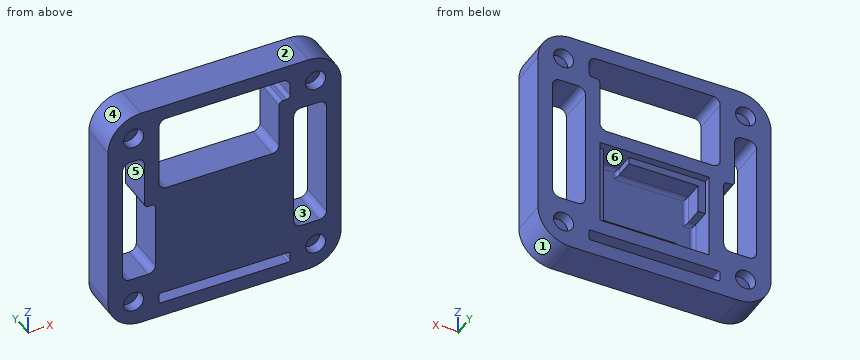
Autodesk Inventor part; units mm, degrees
ref_plane "Work Plane9" through (0, 5, 0) normal (0, 1, 0) x (1, 0, 0)
ref_plane "YZ Plane" through (0, 0, 0) normal (1, 0, 0) x (0, 1, 0)
ref_plane "XZ Plane" through (0, 0, 0) normal (0, 1, 0) x (-1, 0, 0)
sketch "Sketch1" plane through (0, 0, 0) normal (0, 1, 0) x (-1, 0, 0)
  line L0 (30, 30) -> (-30, 30)
  line L1 (-30, 30) -> (-30, -30)
  line L2 (-30, -30) -> (30, -30)
  line L3 (30, -30) -> (30, 30)
  line L4 (30, 30) -> (-30, -30) construction
  line L5 (-30, 30) -> (30, -30) construction
  point P0 (0, 0)
  dimension "d0" = 60
  dimension "d1" = 60
extrude "Extrusion1" add sketch "Sketch1" along normal blind 10
fillet "Fillet1" radius 7 4 edges at (30, 5, 30) (30, 5, -30) (-30, 5, 30) (-30, 5, -30)
sketch "Sketch2" plane through (0, 10, 0) normal (0, 1, 0) x (1, 0, 0)
  line L0 (-30, 30) -> (30, 30)
  line L1 (30, 30) -> (30, -30)
  line L2 (30, -30) -> (-30, -30)
  line L3 (-30, -30) -> (-30, 30)
  line L4 (-30, 30) -> (30, -30) construction
  line L5 (30, 30) -> (-30, -30) construction
  line L6 (25, -25) -> (25, 25)
  line L7 (25, 25) -> (-25, 25)
  line L8 (-25, 25) -> (-25, -25)
  line L9 (-25, -25) -> (25, -25)
  circle A0 centre (25, -25) radius 2.75
  circle A1 centre (-25, -25) radius 2.75
  circle A2 centre (25, 25) radius 2.75
  circle A3 centre (-25, 25) radius 2.75
  point P0 (0, 0)
  dimension "d5" = 5
  dimension "d6" = 5.5
  dimension "d7" = 5.5
  dimension "d8" = 5.5
  dimension "d9" = 5.5
extrude "Extrusion2" cut sketch "Sketch2" against normal blind 3 contours L9 A0 L6 | L6 A0 L9 | A2 L7 L6 | L6 L7 A2 | A1 L8 L9 | L9 L8 A1 | A3 L8 L7 | L7 L8 A3
sketch "Sketch7" plane through (0, 10, 0) normal (0, 1, 0) x (1, 0, 0)
  line L0 (-23, 30) -> (23, 30)
  line L1 (30, 23) -> (30, -23)
  line L2 (23, -30) -> (-23, -30)
  line L3 (-30, -23) -> (-30, 23)
  line L4 (-30, 30) -> (30, -30) construction
  line L5 (30, 30) -> (-30, -30) construction
  arc A0 (-23, 30) -> (-30, 23) centre (-23, 23) ccw
  arc A1 (-30, -23) -> (-23, -30) centre (-23, -23) ccw
  arc A2 (23, -30) -> (30, -23) centre (23, -23) ccw
  arc A3 (30, 23) -> (23, 30) centre (23, 23) ccw
  line L6 (23, 32) -> (-23, 32)
  arc A4 (-23, 32) -> (-32, 23) centre (-23, 23) ccw
  line L7 (-32, 23) -> (-32, -23)
  arc A5 (-32, -23) -> (-23, -32) centre (-23, -23) ccw
  line L8 (-23, -32) -> (23, -32)
  arc A6 (23, -32) -> (32, -23) centre (23, -23) ccw
  line L9 (32, -23) -> (32, 23)
  arc A7 (32, 23) -> (23, 32) centre (23, 23) ccw
  point P0 (0, 0)
  dimension "d47" = 7
  dimension "d48" = 2
extrude "Extrusion6" add sketch "Sketch7" against normal blind 10
sketch "Sketch33" plane through (0, 10, 0) normal (0, 1, 0) x (1, 0, 0)
  line L0 (-25, 25) -> (25, 25)
  line L1 (25, 25) -> (25, -25)
  line L2 (25, -25) -> (-25, -25)
  line L3 (-25, -25) -> (-25, 25)
  line L4 (-25, 25) -> (25, -25) construction
  line L5 (25, 25) -> (-25, -25) construction
  line L6 (21, 21) -> (-21, 21)
  line L7 (-21, 21) -> (-21, -21)
  line L8 (-21, -21) -> (21, -21)
  line L9 (21, -21) -> (21, 21)
  line L10 (-15, 21) -> (-15, -2.8)
  line L11 (-15, -2.8) -> (15, -2.8)
  line L12 (15, -2.8) -> (15, 21)
  line L13 (-13, 7) -> (-13, -0.8)
  line L14 (-13, -0.8) -> (6, -0.8)
  line L15 (13, -0.8) -> (13, 19)
  line L16 (-7, 21) -> (-7, 19)
  line L17 (-7, 19) -> (13, 19)
  line L18 (13, -0.8) -> (13, -2.8)
  line L19 (6, -2.8) -> (6, -0.8)
  line L20 (-15, 7) -> (-13, 7)
  point P0 (0, 0)
  point P1 (-21, 15)
  dimension "d349" = 50
  dimension "d350" = 50
  dimension "d351" = 4
  dimension "d352" = 6
  dimension "d353" = 30
  dimension "d354" = 6
  dimension "d355" = 23.8
  dimension "d356" = 8
  dimension "d357" = 2
  dimension "d358" = 7
  dimension "d359" = 2
  dimension "d360" = 2
  dimension "d361" = 14
extrude "Extrusion31" cut sketch "Sketch33" against normal blind 2 contours L12 L11 L18 L15 L17 L16 L6 | L20 L13 L14 L19 L11 L10
sketch "Sketch34" plane through (0, 10, 0) normal (0, 1, 0) x (1, 0, 0)
  line L0 (13, -2.8) -> (6, -2.8)
  line L1 (6, -2.8) -> (6, -0.8)
  line L2 (6, -0.8) -> (-13, -0.8)
  line L3 (-13, -0.8) -> (-13, 7)
  line L4 (-13, 7) -> (-15, 7)
  line L5 (-15, 7) -> (-15, 21)
  line L6 (-15, 21) -> (-7, 21)
  line L7 (-7, 21) -> (-7, 19)
  line L8 (-7, 19) -> (13, 19)
  line L9 (13, 19) -> (13, -2.8)
  line L10 (13, -2.8) -> (13, 19)
  point P0 (0, 0)
extrude "Extrusion32" cut sketch "Sketch34" against normal blind 8
sketch "Sketch35" plane through (0, 10, 0) normal (0, 1, 0) x (1, 0, 0)
  line L0 (23, 32) -> (-23, 32)
  line L1 (-32, 23) -> (-32, -23)
  line L2 (32, -23) -> (32, 23)
  line L3 (-15, 21) -> (15, 21)
  line L4 (18, 28) -> (-18, 28)
  line L5 (-18, 28) -> (-18, 25)
  line L6 (-18, 25) -> (18, 25)
  line L7 (18, 25) -> (18, 28)
  line L8 (-23, -32) -> (23, -32)
  line L9 (15, 21) -> (15, -2.8)
  line L10 (28, -18) -> (28, 18)
  line L11 (28, 18) -> (19, 18)
  line L12 (19, 18) -> (19, -18)
  line L13 (19, -18) -> (28, -18)
  line L14 (15, -2.8) -> (-15, -2.8)
  line L15 (-18, -28) -> (18, -28)
  line L16 (18, -28) -> (18, -22)
  line L17 (18, -22) -> (15, -22)
  line L18 (15, -22) -> (15, -6.8)
  line L19 (15, -6.8) -> (-18, -6.8)
  line L20 (-18, -6.8) -> (-18, -28)
  line L21 (-15, -2.8) -> (-15, 21)
  line L22 (-22, -18) -> (-28, -18)
  line L23 (-28, -18) -> (-28, 18)
  line L24 (-28, 18) -> (-19, 18)
  line L25 (-19, 18) -> (-19, -2.8)
  line L26 (-19, -2.8) -> (-22, -2.8)
  line L27 (-22, -2.8) -> (-22, -18)
  point P0 (0, 0)
  dimension "d366" = 4
  dimension "d367" = 4
  dimension "d368" = 14
  dimension "d369" = 14
  dimension "d370" = 4
  dimension "d371" = 4
  dimension "d372" = 14
  dimension "d373" = 4
  dimension "d374" = 14
  dimension "d375" = 4
  dimension "d376" = 4
  dimension "d377" = 14
  dimension "d378" = 4
  dimension "d379" = 4
  dimension "d380" = 4
  dimension "d381" = 14
  dimension "d382" = 4
  dimension "d383" = 14
  dimension "d384" = 14
  dimension "d385" = 4
  dimension "d386" = 4
  dimension "d387" = 4
extrude "Extrusion33" cut sketch "Sketch35" against normal through all contours L7 L6 L5 L4 | L13 L12 L11 L10 | L20 L19 L18 L17 L16 L15 | L22 L23 L24 L25 L26 L27
fillet "Fillet10" radius 2 12 edges at (19, 5, 18) (-28, 5, 18) (-18, 5, 28) (15, 5, 6.8) (28, 5, -18) (28, 5, 18) (18, 5, 28) (-18, 5, 6.8) (19, 5, -18) (-28, 5, -18) (-19, 5, -18) (-22, 5, 18)
fillet "Fillet10" radius 1 14 edges at (15, 5, 22) (9.5, 2, 2.8) (13, 2, -8.1) (-3.5, 2, 0.8) (-13, 2, -3.1) (-15, 2, -14) (-22, 5, 2.8) (-19, 5, 2.8) (18, 5, 22) (3, 2, -19) (-11, 2, -21) (-14, 2, -7) (6, 2, 1.8) (-7, 2, -20)
fillet "Fillet10" radius 0.5 4 edges at (-18, 5, -25) (-18, 5, -28) (18, 5, -25) (18, 5, -28)
ref_plane "Work Plane9" through (0, 5, 0) normal (0, 1, 0) x (1, 0, 0)
mirror "Mirror9" about plane through (0, 5, 0) normal (0, 1, 0) of "Extrusion2"
properties part number "8 pinshort"
CAD build for the part. Positions are in the model's coordinates, mm. Face numbers are marked on the shaded views. A direction names the side the tool comes from. Give positions to 0.01 mm unless a question says otherwise; leave off trailing zeros. Write each loop counter-clockwise with the first axis right and the second up, starting at its lowest first coordinate (ties: lowest second). Pieces come first, ordered by that corner, then holes. Notation, with made-up numbers: (39.5, 67) -> (95.5, 67) arc R7 ccw to (95.5, 76) -> close; hole circle Ø5 at (79.5, 47). An arc over 180 degrees is marked (long way). Return JSON: item names as keys, results as strings.
Item 1: Band-saw the part on A-A (x = 3). List the corners of the cut face in (y, z).
Answer below:
{"outline": "(0, -32) -> (10, -32) -> (10, -28) -> (0, -28) -> close; (0, -25) -> (10, -25) -> (10, -21) -> (8, -21) -> (8, -19) -> (3, -19) arc R1 cw to (2, -18) -> (2, -0.2) arc R1 cw to (3, 0.8) -> (8, 0.8) -> (8, 2.8) -> (10, 2.8) -> (10, 6.8) -> (0, 6.8) -> close; (0, 28) -> (10, 28) -> (10, 32) -> (0, 32) -> close"}
Item 2: Two-plate mould, pull along Z, no slides. Class the marked faces 1, 2 and 3: +Z half, -Z half, draft (parallel to the pull), parting line (faces both ways), or undercut.
Answer below:
{"face 1": "-Z half", "face 2": "+Z half", "face 3": "undercut"}
Item 3: Drill centre lines: probe 1 along X at (y, z) = (5, -0.5); probe 2 along Z at (x, y) = (4, 8.75); probe 3 along X at (y, z) = (6.5, 14). Where is each one in solid material? Low to high.
Answer below:
{"probe 1": "x = -32 to -28, -19 to -13, 13 to 19, 28 to 32", "probe 2": "z = -32 to -28, -25 to -21, 2.8 to 6.8, 28 to 32", "probe 3": "x = -32 to -28, -22 to -18, 15 to 19, 28 to 32"}
Item 4: Tool access for the marked faces 4, 5 and 6: list every direction of +Z, -Z, +X, -X, +Y, -Y with a clear straight run to the whole face (end or side of a thin tool).
Answer below:
{"face 4": "+Z, -X, +Y, -Y", "face 5": "+Y, -Y", "face 6": "+Y"}
Item 5: Band-saw the part on C-C (x = -25). List the corners of the cut face in (y, z), then the cut area to 3 significant figures.
Answer below:
{"outline": "(0, -31.77) -> (10, -31.77) -> (10, -27.75) -> (7, -27.75) -> (7, -22.25) -> (10, -22.25) -> (10, -18) -> (0, -18) -> (0, -22.25) -> (3, -22.25) -> (3, -27.75) -> (0, -27.75) -> close; (0, 18) -> (10, 18) -> (10, 22.25) -> (7, 22.25) -> (7, 27.75) -> (10, 27.75) -> (10, 31.77) -> (0, 31.77) -> (0, 27.75) -> (3, 27.75) -> (3, 22.25) -> (0, 22.25) -> close", "area": "209 mm2"}
Item 6: Drop flat-ended pins along their axis: pin 1 (6.5 mm diameter, centred on x = 25, z = -25, fed in from +Y); pin 2 (4.5 mm diameter, centred on x = -25, z = 25, fed in from +Y); pin 3 (1.6 mm diameter, centred on y = 7, z = -26.5, fed in from -X); pin 4 (1.5 mm diameter, centred on x = 24.5, y = 7, fed in from -Z). Give the stop position or say it passes through.
Answer below:
{"pin 1": "stops at y = 10", "pin 2": "stops at y = 7", "pin 3": "stops at x = -31.59", "pin 4": "stops at z = -31.97"}
Item 7: Band-saw the part on B-B (z = 11). List the corners of the cut face in (x, y).
Answer below:
{"outline": "(-32, 0) -> (-28, 0) -> (-28, 10) -> (-32, 10) -> close; (-22, 0) -> (-18, 0) -> (-18, 10) -> (-22, 10) -> close; (15, 0) -> (19, 0) -> (19, 10) -> (15, 10) -> close; (28, 0) -> (32, 0) -> (32, 10) -> (28, 10) -> close"}
Item 8: Band-saw the part on D-D (z = -9.5). List the corners of the cut face in (x, y), then the cut area to 3 significant figures.
Answer below:
{"outline": "(-32, 0) -> (-28, 0) -> (-28, 10) -> (-32, 10) -> close; (-19, 0) -> (19, 0) -> (19, 10) -> (15, 10) -> (15, 8) -> (13, 8) -> (13, 3) arc R1 cw to (12, 2) -> (-14, 2) arc R1 cw to (-15, 3) -> (-15, 10) -> (-19, 10) -> close; (28, 0) -> (32, 0) -> (32, 10) -> (28, 10) -> close", "area": "232 mm2"}
